Work out the finished part from the listing and answer in its coordinate system (mm). A direction names the side the tool comes from. Round coordinates to 2 decimals unless told otherwise and drop trailing zeros. Loops run counter-clockwise (first coordinate to the right, second up) from the corner with the lowest first, then second, coordinate; pieces in that order, holes last. Notation, with made-up numbers: (31, 32) - (88, 32) arc R19 ccw to (88, 58) - close; hole circle Ø11 at (-21, -11.5). An arc over 180 degrees is marked (long way). Use CSV: the item, a comma, the result in double quotes. Start each with the question number.
from build123d import *

# Parameters (mm, degrees)
SKETCH1_W                                           = 125
SKETCH1_H                                           = 60
BOSS_EXTRUDE1_DEPTH                                 = 10
SKETCH12_R                                          = 3
BOSS_EXTRUDE2_DEPTH                                 = 25
M10_TAPPED_HOLE1_D                                  = 8.5
M10_TAPPED_HOLE1_DEPTH                              = 24.5
M10_TAPPED_HOLE1_CSINK_D                            = 10
M10_TAPPED_HOLE1_CSINK_ANGLE                        = 90
M10_TAPPED_HOLE1_TIP                                = 2.553657631
SKETCH7_R                                           = 3.75
CUT_EXTRUDE1_DEPTH                                  = 141.890028036
CBORE_FOR_M3_HEX_SOCKET_HEAD_CAP_SCREW1_D           = 3.4
CBORE_FOR_M3_HEX_SOCKET_HEAD_CAP_SCREW1_CBORE_D     = 7
CBORE_FOR_M3_HEX_SOCKET_HEAD_CAP_SCREW1_CBORE_DEPTH = 5
M5_TAPPED_HOLE1_D                                   = 4.2
M5_TAPPED_HOLE1_DEPTH                               = 12.4
M5_TAPPED_HOLE1_TIP                                 = 1.2618073
CHAMFER2_SIZE                                       = 0.5


with BuildPart() as part:
    # Sketch1 → Boss-Extrude1 (new body)
    with BuildSketch(Plane(origin=(0, 0, 0), x_dir=(0, 0, -1), z_dir=(1, 0, 0))):
        with Locations((-62.5, 30)):
            Rectangle(SKETCH1_W, SKETCH1_H)
    extrude(amount=BOSS_EXTRUDE1_DEPTH)

    # Sketch12 → Boss-Extrude2 (add)
    with BuildSketch(Plane(origin=(10, 0, 0), x_dir=(0, 0, -1), z_dir=(1, 0, 0))):
        with Locations((-55, 10)):
            Circle(SKETCH12_R)
        with Locations((-55, 50)):
            Circle(SKETCH12_R)
    extrude(amount=BOSS_EXTRUDE2_DEPTH)

    # M10 Tapped Hole1
    with Locations(Plane(origin=(10, 0, 0), x_dir=(0, 0, -1), z_dir=(1, 0, 0))):
        with Locations((-115, 30)):
            CounterSinkHole(M10_TAPPED_HOLE1_D / 2, M10_TAPPED_HOLE1_CSINK_D / 2, depth=M10_TAPPED_HOLE1_DEPTH, counter_sink_angle=M10_TAPPED_HOLE1_CSINK_ANGLE)
            with Locations((0, 0, -(M10_TAPPED_HOLE1_DEPTH + M10_TAPPED_HOLE1_TIP / 2))):  # 118° drill point
                Cone(0, M10_TAPPED_HOLE1_D / 2, M10_TAPPED_HOLE1_TIP, mode=Mode.SUBTRACT)

    # Sketch7 → Cut-Extrude1 (cut, through all)
    with BuildSketch(Plane(origin=(10, 0, 0), x_dir=(0, 0, -1), z_dir=(1, 0, 0))):
        with Locations((-12, 30)):
            Circle(SKETCH7_R)
    extrude(amount=-CUT_EXTRUDE1_DEPTH, mode=Mode.SUBTRACT)

    # CBORE for M3 Hex Socket Head Cap Screw1 (through all)
    with Locations(Plane(origin=(10, 0, 0), x_dir=(0, 0, -1), z_dir=(1, 0, 0))):
        with Locations((-70, 20), (-55, 20), (-55, 40), (-70, 40)):
            CounterBoreHole(CBORE_FOR_M3_HEX_SOCKET_HEAD_CAP_SCREW1_D / 2, CBORE_FOR_M3_HEX_SOCKET_HEAD_CAP_SCREW1_CBORE_D / 2, CBORE_FOR_M3_HEX_SOCKET_HEAD_CAP_SCREW1_CBORE_DEPTH)

    # M5 Tapped Hole1
    with Locations(Plane.XY.offset(125)):
        with Locations((5, 20)):
            Hole(M5_TAPPED_HOLE1_D / 2, depth=M5_TAPPED_HOLE1_DEPTH)
            with Locations((0, 0, -(M5_TAPPED_HOLE1_DEPTH + M5_TAPPED_HOLE1_TIP / 2))):  # 118° drill point
                Cone(0, M5_TAPPED_HOLE1_D / 2, M5_TAPPED_HOLE1_TIP, mode=Mode.SUBTRACT)

    # Chamfer2
    chamfer2_edges = [part.edges().sort_by_distance(p)[0] for p in [
        (35, 10, 58),
        (35, 50, 58),
    ]]
    chamfer(chamfer2_edges, length=CHAMFER2_SIZE)


solid = part.part
Item 1: Which of the six approach directions +Z, -Z, +X, -X, +Y, -Y give full straight-line access (tool end or side, diameter ignored) to faces 1 (the cylindrical face through (2.46, 20.07, 68.3)), 2 (the cylindrical face through (7.535, 42.365, 57.58))?
Item 2: A cutting plane is placed at A-A (z = 115). Determine the outline of the cut face in (x, y), plus the area to 3 significant figures.
Item 3: Each of these flat-tipped pins is pushed along its axis until it touches: pin 1 Ø8 at (y, z) = (40, 55) entering from +X; pin 2 Ø6.5 at (y, z) = (20, 55) entering from +X; pin 3 Ø8 at (x, y) = (29, 50) entering from +Z. Where does it stop, or does it pass through?
Item 4: A cutting plane is placed at D-D (z = 12). Determine the outline of the cut face in (x, y), plus the area to 3 significant figures.
Item 5: A cutting plane is placed at B-B (y = 40). Determine the outline of the cut face in (x, z), plus the area to 3 significant figures.
Item 6: The mould has two halves that part along Y. Classify faces 3 (the cylindrical face through (7.54, 43.47, 70.46)), 4 (the flat face through (5, 0, 63)), 5 (the flat face through (0, 30, 63)): pulls with the +Y half, pulls with the -Y half, needs draft (parallel to the pull), parting line crosses it, or undercut.
Item 7: Find the intervals of material crossed by probe 1 along Y at (x, z) = (7.4, 55); probe 2 along Y at (x, z) = (2.8, 55); probe 3 along X at (y, z) = (20, 119), in increasing order. Write a range as [from, to].
Item 8: A cutting plane is placed at C-C (z = 55). State how many separate pieces and enclosed holes the cut face has, plus the area to 4 significant figures.
Result sheet:
1,face 1,"+X, -X"
1,face 2,"+X"
2,outline,"(0, 0) - (10, 0) - (10, 25) - (9.25, 25.75) - (0, 25.75) - close; (0, 34.25) - (9.25, 34.25) - (10, 35) - (10, 60) - (0, 60) - close; hole circle Ø4.2 at (5, 20)"
2,area,"501 mm^2"
3,pin 1,"x = 10"
3,pin 2,"x = 5"
3,pin 3,"z = 58"
4,outline,"(0, 0) - (10, 0) - (10, 26.25) - (0, 26.25) - close; (0, 33.75) - (10, 33.75) - (10, 60) - (0, 60) - close"
4,area,"525 mm^2"
5,outline,"(0, 0) - (10, 0) - (10, 51.5) - (5, 51.5) - (5, 53.3) - (0, 53.3) - close; (0, 56.7) - (5, 56.7) - (5, 58.5) - (10, 58.5) - (10, 66.5) - (5, 66.5) - (5, 68.3) - (0, 68.3) - close; (0, 71.7) - (5, 71.7) - (5, 73.5) - (10, 73.5) - (10, 125) - (0, 125) - close"
5,area,"1,150 mm^2"
6,face 3,"undercut"
6,face 4,"pulls with the -Y half"
6,face 5,"needs draft"
7,probe 1,"[0, 16.5], [23.5, 36.5], [43.5, 60]"
7,probe 2,"[0, 18.3], [21.7, 38.3], [41.7, 60]"
7,probe 3,"[0, 2.9], [7.1, 10]"
8,separate pieces,"3"
8,enclosed holes,"0"
8,area,"795.5 mm^2"
